Design review of the part shown in the three views and the two pictorial views. Dimensions are in mm from the part's minimum x, y and z. A direction names the side the tool comes from. Coordinates: 2 decimals unless noted, no trailing zeros. Loops run counter-clockwise (first coordinate to the right, second up) from the corner with the lowest first, then second, coordinate; pieces in that order, holes last. Notation, with made-up numbers: (78.5, 82.5) -> (126.5, 82.5) arc R27 cw to (126.5, 111.5) -> close; hole circle Ø2 at (59.25, -40). An arc over 180 degrees is marked (long way). Use CSV: the item, a comma, the result in double quotes.
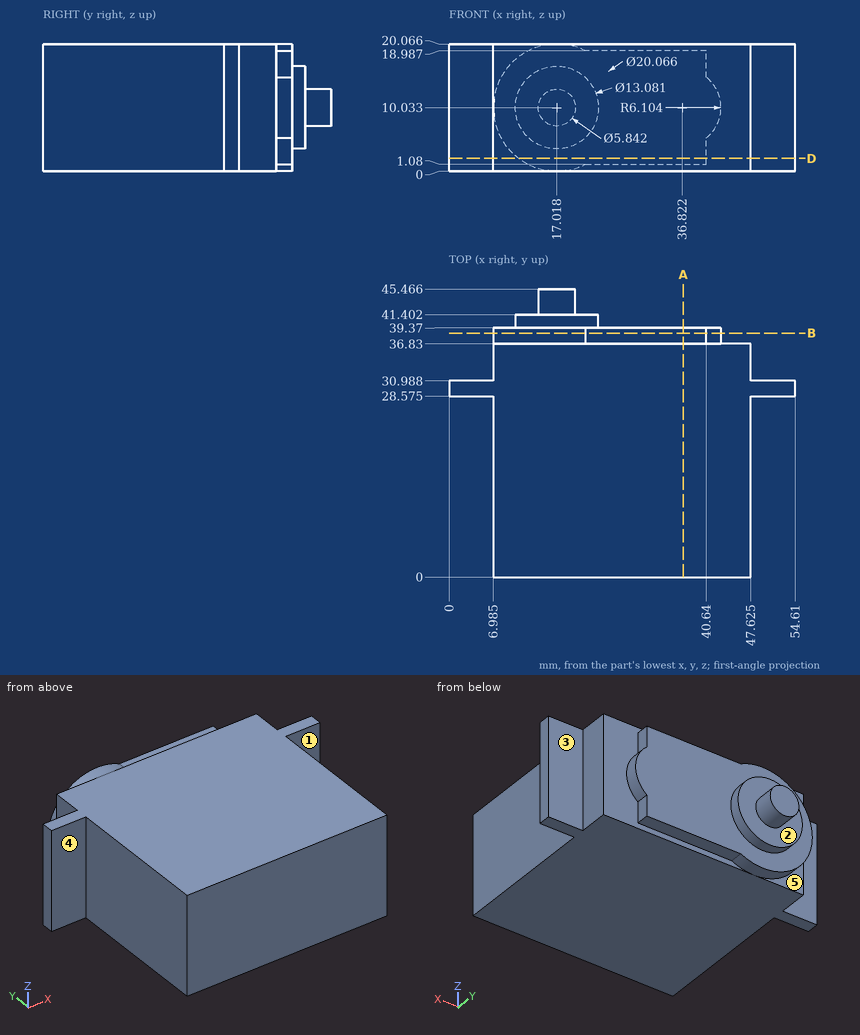
Item 1: Add section D-D (z = 2). Give the boundary of the cut face in (x, y) (1 decimal), then the cut area to 3 significant figures.
Checked values:
outline,"(0, 28.6) -> (7, 28.6) -> (7, 0) -> (47.6, 0) -> (47.6, 28.6) -> (54.6, 28.6) -> (54.6, 31) -> (47.6, 31) -> (47.6, 36.8) -> (40.6, 36.8) -> (40.6, 39.4) -> (11, 39.4) -> (11, 36.8) -> (7, 36.8) -> (7, 31) -> (0, 31) -> close"
area,"1,610 mm^2"
Item 2: Machinability: for the marked faces 1, 2, 3, 4 and 5, which of the approach directions +Z, -Z, +X, -X, +Y, -Y give a long, thin tool a straight path to every point of the face, cutting with its end or side? Answer none if there is none.
Checked values:
face 1,"+Z, -Z, +X, -Y"
face 2,"+Y"
face 3,"+Z, -Z, +X, +Y"
face 4,"+Z, -Z, -X, -Y"
face 5,"-Z, -X, +Y"
Item 3: To check wall thickness, follow line 1 along X through (y, z) = (16.5, 3.5) (1 decimal); line 2 along Y through (x, z) = (35.5, 4.25); line 3 along X through (y, z) = (39.5, 9.75). State the ranges of each line that lie inside material, in increasing order.
Checked values:
line 1,"7 to 47.6"
line 2,"0 to 39.37"
line 3,"10.48 to 23.55"
Item 4: Clearance check with flat-ended pins moving along their axes: pin 1 (10 mm diameter, centred on y = 12.5, z = 12.5, fed in from +X) (1 decimal); pin 2 (2 mm diameter, centred on x = 26.5, y = 38, fed in from +Z); pin 3 (5 mm diameter, centred on x = 45.5, z = 13, fed in from +Y). State where each tip first meets the part, or that it passes through.
Checked values:
pin 1,"x = 47.6"
pin 2,"z = 18.99"
pin 3,"y = 36.83"
Item 5: Add section B-B (y = 38.5). Give the boundary of the cut face in (x, z) (1 decimal), then the cut area to 3 significant figures.
Checked values:
outline,"(21.5, 1.1) -> (40.6, 1.1) -> (40.6, 5.3) arc R6.1 ccw to (40.6, 14.8) -> (40.6, 19) -> (21.5, 19) arc R10 ccw (long way) to start"
area,"603 mm^2"
Item 6: Add section A-A (x = 37). Give the boundary of the cut face in (y, z) (1 decimal).
Checked values:
outline,"(0, 0) -> (36.8, 0) -> (36.8, 1.1) -> (39.4, 1.1) -> (39.4, 19) -> (36.8, 19) -> (36.8, 20.1) -> (0, 20.1) -> close"
